For this review, take the finished solid that the model builds, in its own axes (mm). Face numbers are marked on the shaded views. A direction names the side the tool comes from. Give positions to 0.01 mm unless a question says otherwise; leave off trailing zeros. Write each loop counter-clockwise with the first axis right and the second up, starting at its lowest first coordinate (ties: lowest second). Pieces come first, ordered by that corner, then holes. Notation, with made-up numbers: M 15,57 L 65,57 A27 cw 65,74 Z; hole C 68.5,76 d3. An arc over 180 degrees is marked long. Use one line per item in the form item = value. Start each with the question number.
Q1. Clearance check with flat-ended pins moving along their axes: pin 1 Ø1 at (y, z) = (2, -7) entering from +X; pin 2 Ø2 at (x, z) = (2.5, -4.5) entering from -Y; pin 3 Ø1.5 at (x, y) = (5.5, 2) entering from -Z. State where each tip first meets the part, or that it passes through.
Q2. Tool access review of the marked faces 1, 2 and 3: name each direction out of +Z, -Z, +X, -X, +Y, -Y from which nothing blocks a thin tool from reaching the whole face with its end or side.
Q3. Consider section D-D on z = -2.5. Write out the cut boundary in (x, y), and give its area (3 significant figures).
Q4. Consider section A-A on z = -4.25. Write out the cut boundary in (x, y), and give its area (3 significant figures).
Q5. Mouldability with a two-part tool opening along Z and no side actions: class the marked faces 4, 5 and 6 as released by +Z, released by -Z, zero draft, split by the parting line, or undercut.
Q6. Consider section C-C on y = 1.95. Write out the cut boundary in (x, z), and give its area (3 significant figures).
Q7. Consider section B-B on x = 4. Write out the cut boundary in (y, z), and give its area (3 significant figures).
Q8. For probe 1 along Y at (x, z) = (3.5, -1.75); probe 2 along X at (y, z) = (0.25, -3.75); probe 3 along X at (y, z) = (0.05, -3.5), list the stretches that pass through material, from the lowest coordinate up. Write a range as [from, to].
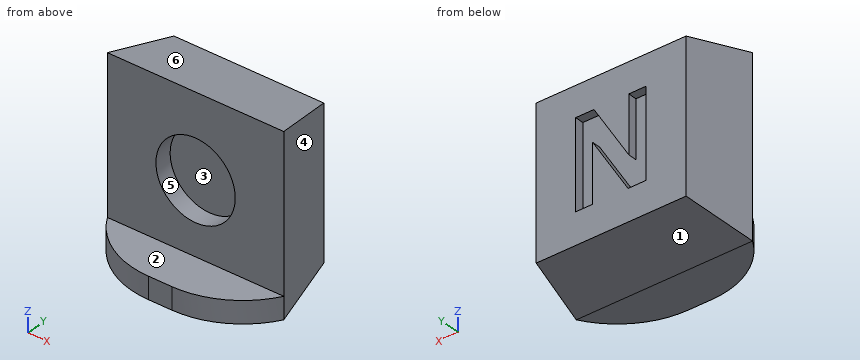
```python
from build123d import *

# Parameters (mm, degrees)
SKETCH1_W               = 8
SKETCH1_H               = 8
BOSS_EXTRUDE1_DEPTH     = 3
CUT_EXTRUDE1_DEPTH      = 12.704699911
CUT_EXTRUDE1_DEPTH_BACK = 12.704699911
CUT_EXTRUDE2_DEPTH      = 11
SKETCH4_R               = 1.8
CUT_EXTRUDE3_DEPTH      = 0.8
SKETCH5_W               = 8
SKETCH5_H               = 1
BOSS_EXTRUDE2_DEPTH     = 2
FILLET1_R               = 4
CUT_EXTRUDE4_DEPTH      = 0.4


with BuildPart() as part:
    # Sketch1 → Boss-Extrude1 (new body)
    with BuildSketch(Plane(origin=(0, 0, 0), x_dir=(1, 0, 0), z_dir=(0, 1, 0))):
        with Locations((4, 4)):
            Rectangle(SKETCH1_W, SKETCH1_H)
    extrude(amount=BOSS_EXTRUDE1_DEPTH)

    # Sketch2 → Cut-Extrude1 (cut, two sides: drawn at the far end of the back side and taken through both)
    with BuildSketch(Plane.XY.offset(-CUT_EXTRUDE1_DEPTH_BACK)):
        Polygon((0, 0), (0.6, 3), (0, 3), align=None)
        Polygon((8, 0), (7.4, 3), (8, 3), align=None)
    extrude(amount=CUT_EXTRUDE1_DEPTH + CUT_EXTRUDE1_DEPTH_BACK, mode=Mode.SUBTRACT)

    # Sketch3 → Cut-Extrude2 (cut)
    with BuildSketch(Plane(origin=(0, 0, 0), x_dir=(0, 0, -1), z_dir=(1, 0, 0))):
        Polygon((0, 0), (0.6, 3), (0, 3), align=None)
        Polygon((8, 3), (7.4, 3), (8, 0), align=None)
    extrude(amount=CUT_EXTRUDE2_DEPTH, mode=Mode.SUBTRACT)

    # Sketch4 → Cut-Extrude3 (cut)
    with BuildSketch(Plane.XZ):
        with Locations(Location((4, -3.75, 0), (0, 0, 270))):
            Circle(SKETCH4_R)
    extrude(amount=-CUT_EXTRUDE3_DEPTH, mode=Mode.SUBTRACT)

    # Sketch5 → Boss-Extrude2 (add)
    with BuildSketch(Plane.XZ):
        with Locations((4, -7.5)):
            Rectangle(SKETCH5_W, SKETCH5_H)
    extrude(amount=BOSS_EXTRUDE2_DEPTH)

    # Fillet1
    # the kernel refuses this fillet: 4 mm, written as the material it takes off along each edge
    with BuildSketch(Plane(origin=(8, -2, -16.660254038), x_dir=(0, 1, 0), z_dir=(0, 0, 1)), Plane(origin=(0, -2, 1.660254038), x_dir=(0, 1, 0), z_dir=(0, 0, -1))) as fillet1_piece_1:
        with BuildLine():
            CenterArc((4, 3.464101615), FILLET1_R, 180, 60)
            Line((0, 3.464101615), (-0.08, 3.464101615))
            Line((-0.08, 3.464101615), (-0.08, 0))
            Line((-0.08, 0), (0, -0.08))
            ThreePointArc((0, -0.08), (1, -0.08), (1.96, -0.069282032))
            Line((1.96, -0.069282032), (2, 0))
        make_face()
    extrude(amount=18.320508076, mode=Mode.SUBTRACT)

    # Sketch6 → Cut-Extrude4 (cut)
    with BuildSketch(Plane(origin=(0, 3, 0), x_dir=(1, 0, 0), z_dir=(0, 1, 0))):
        Polygon((2.428562008, 1.972012859), (2.428562008, 5.972012859), (3.232247906, 5.972012859), (4.838818418, 3.342205167), (4.838818418, 5.972012859), (5.608049188, 5.972012859), (5.608049188, 1.972012859), (4.779523547, 1.972012859), (3.197792777, 4.560153885), (3.197792777, 1.972012859), align=None)
    extrude(amount=-CUT_EXTRUDE4_DEPTH, mode=Mode.SUBTRACT)


solid = part.part
```
Working result:
q1.pin_1 = 7.7
q1.pin_2 = 0
q1.pin_3 = -7.75
q2.face_1 = -Z, +X, -X, +Y
q2.face_2 = +Z, +X, -X, -Y
q2.face_3 = -Y
q3.outline = M 0,0 L 2.7,0 L 2.7,0.8 L 5.3,0.8 L 5.3,0 L 8,0 L 7.4,3 L 5.61,3 L 5.61,2.6 L 4.46,2.6 L 4.46,3 L 3.2,3 L 3.2,2.6 L 2.43,2.6 L 2.43,3 L 0.6,3 Z
q3.area = 19.4 mm²
q4.outline = M 0,0 L 2.27,0 L 2.27,0.8 L 5.73,0.8 L 5.73,0 L 8,0 L 7.4,3 L 5.61,3 L 5.61,2.6 L 4.84,2.6 L 4.84,3 L 4.28,3 L 4.28,2.6 L 3.39,2.6 L 3.39,3 L 3.2,3 L 3.2,2.6 L 2.43,2.6 L 2.43,3 L 0.6,3 Z
q4.area = 18.5 mm²
q5.face_4 = zero draft
q5.face_5 = undercut
q5.face_6 = released by +Z
q6.outline = M 0.39,-7.61 L 7.61,-7.61 L 7.61,-0.39 L 0.39,-0.39 Z
q6.area = 52.1 mm²
q7.outline = M -2,-8 L 0,-8 L 3,-7.4 L 3,-4.72 L 2.6,-4.72 L 2.6,-3.25 L 3,-3.25 L 3,-0.6 L 0,0 L 0,-1.95 L 0.8,-1.95 L 0.8,-5.55 L 0,-5.55 L 0,-7 L -2,-7 Z
q7.area = 20.7 mm²
q8.probe_1 = [0, 3]
q8.probe_2 = [0.05, 2.2], [5.8, 7.95]
q8.probe_3 = [0.01, 2.22], [5.78, 7.99]
